Input: part model. Units: mm. Frame: model coordinates. Face numbers are marked on the shaded views. Coordinates: 2 decimals unless noted, no trailing zeros. Order: outer loops, then holes, each group sorted by start corner. A loop starts at its lowest first (then second) coordinate and runs counter-clockwise, first axis right, second up. Notation, with made-up numbers: (5.25, 43) -> (23.25, 43) arc R18 ccw to (23.25, 72) -> close; hole circle Ø3 at (-23, 74.25). An arc over 180 degrees is marked (long way). One line per item, written item: value. Start each with the question number.
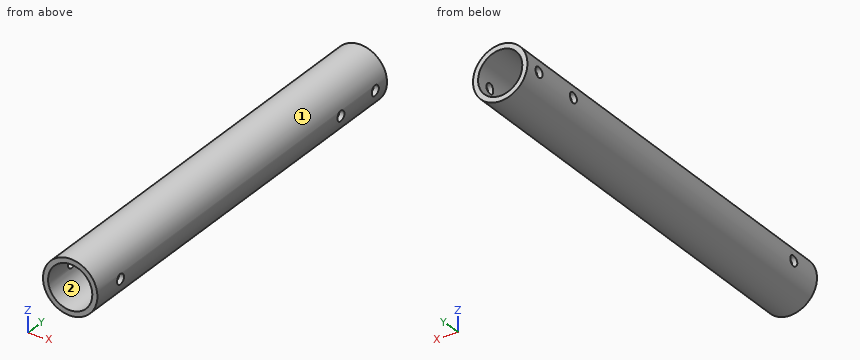
from build123d import *

# Parameters (mm, degrees)
SKETCH_1_R          = 8
SKETCH_1_R_2        = 6.5
EXTRUDE_1_DEPTH     = 125
SKETCH_3_R          = 1.5
CUT_EXTRUDE_2_DEPTH = 62.5


with BuildPart() as part:
    # 草图1 → 凸台-拉伸1 (new body)
    with BuildSketch(Plane(origin=(0, 0, 0), x_dir=(1, 0, 0), z_dir=(0, 1, 0))):
        with Locations(Location((0, 0, 0), (0, 0, 270))):
            Circle(SKETCH_1_R)
        with Locations(Location((0, 0, 0), (0, 0, 270))):
            Circle(SKETCH_1_R_2, mode=Mode.SUBTRACT)
    extrude(amount=EXTRUDE_1_DEPTH)

    # 草图3 → 切除-拉伸2 (cut, symmetric)
    with BuildSketch(Plane(origin=(0, 0, 0), x_dir=(0, 0, -1), z_dir=(1, 0, 0))):
        with Locations((0, 119.968615881)):
            Circle(SKETCH_3_R)
        with Locations((0, 105.132120497)):
            Circle(SKETCH_3_R)
        with Locations((0, 10)):
            Circle(SKETCH_3_R)
    extrude(amount=CUT_EXTRUDE_2_DEPTH, both=True, mode=Mode.SUBTRACT)


solid = part.part
1) Mould query, pull axis Z, two halves, no side actions, for the marked faces 1 and 2. Classes: +Z half, -Z half, draft (parallel to the pull), parting line (faces both ways), or undercut.
2) Section query C-C, the plane y = 10. Return the cut outline in (x, z).
3) Section query B-B, the plane z = 0. State how many separate pieces and enclosed holes the cut face has, plus the area to 3 significant figures.
4) Pin query (flat end, axial travel): pin 1 Ø2.5 at (y, z) = (10, 0) entering from +X (1 decimal); pin 2 Ø6 at (y, z) = (78, 4) entering from +X; pin 3 Ø4 at (x, y) = (4.5, 81) entering from -Z; pin 4 Ø3 at (x, y) = (-6, 37) entering from -Z. Return the tip coordinate at first contact, or that it passes through.
5) Ray query, line 1 along Y through (x, z) = (7, 0); line 2 along Z through (x, y) = (-2.5, 119); line 3 along X through (y, z) = (113, -5.25). Return the intervals inside material, ascending. Write a range as from..to.
6) Section query D-D, the plane y = 43.5. Return the cut outline in (x, z), plus the area to 3 significant figures.
7) Section query A-A, the plane x = 0. Return the cut outline in (y, z), plus the area to 3 significant figures.
Entries:
1. face 1: parting line
1. face 2: undercut
2. outline: (-7.86, -1.5) arc R8 ccw to (7.86, -1.5) -> (6.32, -1.5) arc R6.5 cw to (-6.32, -1.5) -> close; (-7.86, 1.5) -> (-6.32, 1.5) arc R6.5 cw to (6.32, 1.5) -> (7.86, 1.5) arc R8 ccw to start
3. separate pieces: 8
3. enclosed holes: 0
3. area: 348 mm2
4. pin 1: passes through
4. pin 2: stops at x = 7.94
4. pin 3: stops at z = -7.6
4. pin 4: stops at z = -6.61
5. line 1: y = 0..8.5, 11.5..103.63, 106.63..118.47, 121.47..125
5. line 2: z = -7.6..-6, 6..7.6
5. line 3: x = -6.04..-3.83, 3.83..6.04
6. outline: circle Ø16 at (0, 0); hole circle Ø13 at (0, 0)
6. area: 68.3 mm2
7. outline: (0, -8) -> (125, -8) -> (125, -6.5) -> (0, -6.5) -> close; (0, 6.5) -> (125, 6.5) -> (125, 8) -> (0, 8) -> close
7. area: 375 mm2
